Autodesk Inventor part; units mm, degrees
ref_plane "YZ Plane" through (0, 0, 0) normal (1, 0, 0) x (0, 1, 0)
ref_plane "XZ Plane" through (0, 0, 0) normal (0, 1, 0) x (-1, 0, 0)
ref_plane "XY Plane" through (0, 0, 0) normal (0, 0, 1) x (1, 0, 0)
sketch "スケッチ8" plane through (0, 0, 0) normal (0, 1, 0) x (-1, 0, 0)
  line L0 (0, 0) -> (48.6, 0)
  line L1 (48.6, 0) -> (48.6, 32.6)
  line L2 (48.6, 32.6) -> (0, 32.6)
  line L3 (0, 32.6) -> (0, 0)
  circle A0 centre (5.3, 27.3) radius 1.5
  circle A1 centre (43.3, 27.3) radius 1.5
  circle A2 centre (8.3, 3.6) radius 1.5
  circle A3 centre (40.3, 3.6) radius 1.5
  circle A4 centre (24.3, 24.3) radius 5
  line L4 (19.3, 24.3) -> (29.3, 24.3)
  line L5 (29.3, 24.3) -> (29.3, 32.6)
  line L6 (29.3, 32.6) -> (19.3, 32.6)
  line L7 (19.3, 32.6) -> (19.3, 24.3)
  line L8 (0, 32.6) -> (48.6, 32.6)
  line L9 (48.6, 32.6) -> (48.6, 36.8)
  line L10 (48.6, 36.8) -> (0, 36.8)
  line L11 (0, 36.8) -> (0, 32.6)
  arc A5 (11.9042, 0) -> (36.6958, 0) centre (24.3, 10.7) ccw
  arc A6 (29.3, 25.8987) -> (29.0048, 25.9926) centre (24.3, 10.7) ccw
  arc A7 (19.5952, 25.9926) -> (19.3, 25.8987) centre (24.3, 10.7) ccw
  line L12 (11.9042, 0) -> (36.6958, 0)
  dimension "d42" = 32.6
  dimension "d43" = 48.6
  dimension "d44" = 3
  dimension "d45" = 3
  dimension "d46" = 3
  dimension "d47" = 3
  dimension "d48" = 38
  dimension "d49" = 32
  dimension "d50" = 5.3
  dimension "d51" = 8.3
  dimension "d52" = 5.3
  dimension "d53" = 0
  dimension "d54" = 3.6
  dimension "d55" = 0
  dimension "d56" = 10
  dimension "d57" = 19
  dimension "d58" = 8.3
  dimension "d61" = 36.8
  dimension "d103" = 10.7
  dimension "d104" = 0
extrude "押し出し8" add sketch "スケッチ8" along normal blind 2 contours L3 L2 L7 A4 L5 L1 L0 | L0 A5
fillet "フィレット3" radius 10 4 edges at (0, 1, 32.6) (0, 1, 0) (-48.6, 1, 0) (-48.6, 1, 32.6)
sketch "スケッチ9" plane through (0, 0, 0) normal (0, -1, 0) x (1, 0, 0)
  line L0 (-10, 0) -> (-38.6, 0)
  line L1 (-48.5604, 35.5868) -> (6.5479, 35.5868)
  line L2 (6.5479, 35.5868) -> (6.5479, 31.8)
  line L3 (6.5479, 31.8) -> (-48.5604, 31.8)
  line L4 (-48.5604, 31.8) -> (-48.5604, 35.5868)
  point P0 (0, 0)
  dimension "d63" = 31.8
extrude "押し出し9" cut sketch "スケッチ9" against normal blind 2
sketch "スケッチ10" plane through (0, 0, 0) normal (0, -1, 0) x (1, 0, 0)
  arc A0 (-29.3, 24.3) -> (-19.3, 24.3) centre (-24.3, 24.3) ccw
  line L0 (-47.1, 20.3) -> (-45.8, 20.3)
  line L1 (-45.8, 20.3) -> (-45.8, 11)
  line L2 (-45.8, 11) -> (-47.1, 11)
  line L3 (-47.1, 11) -> (-47.1, 20.3)
  line L4 (-47.1, 11) -> (-39.8, 11)
  line L5 (-39.8, 11) -> (-39.8, 12.3)
  line L6 (-39.8, 12.3) -> (-47.1, 12.3)
  line L7 (-47.1, 12.3) -> (-47.1, 11)
  line L8 (-1.5, 20.3) -> (-2.8, 20.3)
  line L9 (-2.8, 20.3) -> (-2.8, 11)
  line L10 (-2.8, 11) -> (-1.5, 11)
  line L11 (-1.5, 11) -> (-1.5, 20.3)
  line L12 (-1.5, 11) -> (-8.8, 11)
  line L13 (-8.8, 11) -> (-8.8, 12.3)
  line L14 (-8.8, 12.3) -> (-1.5, 12.3)
  line L15 (-1.5, 12.3) -> (-1.5, 11)
  point P0 (0, 0)
  dimension "d66" = 43
  dimension "d67" = 21.5
  dimension "d68" = 1.3
  dimension "d69" = 1.3
  dimension "d70" = 1.3
  dimension "d71" = 1.3
  dimension "d72" = 0
  dimension "d73" = 8
  dimension "d74" = 8
  dimension "d75" = 12
  dimension "d76" = 6
  dimension "d77" = 6
extrude "押し出し10" add sketch "スケッチ10" along normal blind 1.5
sketch "スケッチ11" plane through (0, -1.5, 0) normal (0, -1, 0) x (1, 0, 0)
  line L0 (-45.8, 12.3) -> (-45.8, 20.3)
  line L1 (-45.8, 20.3) -> (-47.1, 20.3)
  line L2 (-47.1, 20.3) -> (-47.1, 11)
  line L3 (-47.1, 11) -> (-39.8, 11)
  line L4 (-39.8, 11) -> (-39.8, 12.3)
  line L5 (-39.8, 12.3) -> (-45.8, 12.3)
  line L6 (-47.1, 11) -> (-39.8, 11)
  line L7 (-39.8, 11) -> (-39.8, 20.3)
  line L8 (-39.8, 20.3) -> (-47.1, 20.3)
  line L9 (-47.1, 20.3) -> (-47.1, 11)
  line L10 (-1.5, 11) -> (-8.8, 11)
  line L11 (-8.8, 11) -> (-8.8, 20.3)
  line L12 (-8.8, 20.3) -> (-1.5, 20.3)
  line L13 (-1.5, 20.3) -> (-1.5, 11)
  point P0 (0, 0)
extrude "押し出し11" add sketch "スケッチ11" along normal blind 1.3
sketch "スケッチ12" plane through (0, -2.8, 0) normal (0, -1, 0) x (1, 0, 0)
  line L0 (-47.1, 11) -> (-39.8, 11)
  line L1 (-39.8, 11) -> (-39.8, 20.3)
  line L2 (-39.8, 20.3) -> (-47.1, 20.3)
  line L3 (-47.1, 20.3) -> (-47.1, 11)
  circle A0 centre (-41.8, 16.3) radius 1.5
  circle A1 centre (-6.8, 16.3) radius 1.5
  arc A2 (-29.3, 24.3) -> (-19.3, 24.3) centre (-24.3, 24.3) ccw
  point P0 (0, 0)
  dimension "d82" = 3
  dimension "d83" = 3
  dimension "d84" = 35
  dimension "d85" = 17.5
  dimension "d86" = 0
  dimension "d87" = 8
extrude "押し出し12" cut sketch "スケッチ12" against normal blind 10 contours A0 | A1
chamfer "面取り3" distance 1.2 distance2 7 1 edges at (-39.8, -2.15, 20.3) measured on face at (-39.8, -2.3667, 14.5333)
chamfer "面取り4" distance 1.2 distance2 7 1 edges at (-8.8, -2.15, 20.3) measured on face at (-8.8, -2.3667, 14.5333)
chamfer "面取り5" distance 1.2 angle 45 2 edges at (-43.3, -2.8, 19.7) (-5.3, -2.8, 19.7)
sketch "スケッチ14" plane through (-19.3, 0, 31.8) normal (0, 0, 1) x (1, 0, 0)
  line L0 (13.2192, 0) -> (0, 0)
  line L1 (0, 2) -> (13.2192, 2)
  line L2 (-10, 2) -> (-10, 0)
  line L3 (-23.2192, 2) -> (-10, 2)
  line L4 (-23.2192, 0) -> (-23.2192, 2)
  line L5 (-10, 0) -> (-23.2192, 0)
  line L6 (-15.5703, 7) -> (-14.5703, 7)
  line L7 (-14.5703, 7) -> (-14.5703, -5)
  line L8 (-14.5703, -5) -> (-15.5703, -5)
  line L9 (-15.5703, -5) -> (-15.5703, 7)
  line L10 (6.2462, 7) -> (7.2462, 7)
  line L11 (7.2462, 7) -> (7.2462, -5)
  line L12 (7.2462, -5) -> (6.2462, -5)
  line L13 (6.2462, -5) -> (6.2462, 7)
  point P0 (19.3, 0)
  dimension "d114" = 1
  dimension "d115" = 1
  dimension "d116" = 5
  dimension "d117" = 5
  dimension "d118" = 5
  dimension "d119" = 5
extrude "押し出し14" add sketch "スケッチ14" against normal blind 7 contours L11 L12 L13 L0 | L0 L13 L1 L11 | L1 L13 L10 L11 | L7 L5 L9 L3 | L3 L9 L6 L7 | L7 L8 L9 L5
chamfer "面取り6" distance 5 distance2 7 1 edges at (-12.5538, -5, 24.8) measured on face at (-12.7204, -1.6667, 24.8)
chamfer "面取り7" distance 5 distance2 7 1 edges at (-34.3703, -5, 24.8) measured on face at (-34.5369, -1.6667, 24.8)
chamfer "面取り8" distance 5 distance2 7 1 edges at (-12.5538, 7, 24.8) measured on face at (-12.7204, 5.3333, 24.8)
chamfer "面取り9" distance 5 distance2 7 1 edges at (-34.3703, 7, 24.8) measured on face at (-34.5369, 5.3333, 24.8)
fillet "フィレット5" radius 1 2 edges at (-42.8, -1.5, 12.3) (-5.8, -1.5, 12.3)
equation "\"d45\" = d44"
equation "\"d46\" = d44"
equation "\"d47\" = d44"
equation "\"d57\" = 0.5 * d48"
equation "\"d67\" = 0.5 * d66"
equation "\"d69\" = d68"
equation "\"d70\" = d68"
equation "\"d71\" = d70"
equation "\"d74\" = d73"
equation "\"d77\" = d76"
equation "\"d83\" = d82"
equation "\"d85\" = 0.5 * d84"
equation "\"d115\" = d114"
equation "\"d117\" = d116"
equation "\"d118\" = d117"
equation "\"d119\" = d116"
properties part number "motor-holder"
The model under review builds one solid part; all positions refer to its coordinate system, in mm. A direction names the side the tool comes from. Round coordinates to 2 decimals unless told otherwise and drop trailing zeros. Order: outer loops, then holes, each group sorted by start corner. A loop starts at its lowest first (then second) coordinate and runs counter-clockwise, first axis right, second up. Notation, with made-up numbers: (76.25, 43) -> (90.25, 43) arc R24 ccw to (90.25, 70) -> close; hole circle Ø9 at (54, 18). An arc over 180 degrees is marked (long way). Use CSV: the item, a comma, the result in double quotes. Start each with the question number.
(1) Consider section A-A on y = 3.25. Write out the cut boundary in (x, z), and give its area (3 significant figures).
(2) Consider section B-B on z = 16.3. State how many separate pieces and enclosed holes the cut face has, and give its area (3 significant figures).
(3) Wall thickness on probe 1 along Y at (x, z) = (-41, 18); probe 2 along Z at (x, y) = (-8, 1.25); probe 3 along X at (y, z) = (-0.25, 12.5): over which ranges is each line inside the solid? List them lowest first. Write a range as from..to.
(4) Tool access review of faces 1 (the face through (-38, 1, 0)), 2 (the face through (-34.87, 4, 29)), 3 (the face through (-5, -1.5, 17)): name each direction out of +Z, -Z, +X, -X, +Y, -Y from which nothing blocks a thin tool from reaching the whole face with its end or side.
(5) Mouldability with a two-part tool opening along X and no side actions: class faces 4 (the face through (-33.87, -2, 29)), 5 (the face through (-46.987, 1.014, 28.046)), 6 (the face through (-5, -1, 11)) as pulls with the +X half, pulls with the -X half, needs draft (parallel to the pull), parting line crosses it, or undercut.
(6) Consider section D-D on z = 3.6. Write out the cut boundary in (x, y), and give its area (3 significant figures).
(7) Insertion check: pin 1 (8 mm diameter, centred on x = -8.5, z = 10, fed in from -Y); pin 2 (0.6 mm diameter, centred on x = -10.5, y = 1, fed in from -Z); pin 3 (1.4 mm diameter, centred on y = -1, z = 16.5, fed in from +X); pin 4 (5 mm diameter, centred on y = 0.5, z = 25, fed in from -X). Each pin has a flat end and moves straight along its axis. Give the tip position at first contact, or say it passes through.
Responses:
1,outline,"(-34.87, 26.55) -> (-33.87, 26.55) -> (-33.87, 31.8) -> (-34.87, 31.8) -> close; (-13.05, 26.55) -> (-12.05, 26.55) -> (-12.05, 31.8) -> (-13.05, 31.8) -> close"
1,area,"10.5 mm²"
2,separate pieces,"5"
2,enclosed holes,"0"
2,area,"100 mm²"
3,probe 1,"-2.8..-1.5, 0..2"
3,probe 2,"0.2..2.13, 5.07..15.4, 17.2..31.8"
3,probe 3,"-47.1..-45.8, -2.8..-1.5"
4,face 1,"-Z, -X, +Y, -Y"
4,face 2,"+Z, -Z, -X, +Y"
4,face 3,"+Z"
5,face 4,"undercut"
5,face 5,"pulls with the -X half"
5,face 6,"needs draft"
6,outline,"(-46.28, 0) -> (-41.8, 0) -> (-41.8, 2) -> (-46.28, 2) -> close; (-38.8, 0) -> (-9.8, 0) -> (-9.8, 2) -> (-38.8, 2) -> close; (-6.8, 0) -> (-2.32, 0) -> (-2.32, 2) -> (-6.8, 2) -> close"
6,area,"75.9 mm²"
7,pin 1,"y = -2.8"
7,pin 2,"z = 0"
7,pin 3,"x = -1.5"
7,pin 4,"x = -48.6"
